Solid Edge part; units mm, degrees
sketch "Sketch1" plane through (0, 0, 0) normal (0, 0, 1) x (1, 0, 0)
  line L0 (-9, 9) -> (9, 9)
  line L1 (9, 9) -> (9, -9)
  line L2 (9, -9) -> (-9, -9)
  line L3 (-9, -9) -> (-9, 9)
  dimension "D1" = 9
  dimension "D2" = 9
extrude "Protrusion1" add sketch "Sketch1" along normal mid plane 6.5
sketch "Sketch2" plane through (0, 0, 3.25) normal (0, 0, 1) x (1, 0, 0)
  circle A0 centre (0, 0) radius 5
extrude "ExtrudedProtrusion_2" add sketch "Sketch2" along normal blind 75
chamfer "Chamfer_1" distance 1 angle 45 1 edges at (-5, 0, 78.25)
cosmetic_thread "Thread_1" thread depth 26
sketch "Sketch3" plane through (0, 0, 0) normal (1, 0, 0) x (0, 1, 0)
  line L0 (9, -3.25) -> (38.1568, 13.5837)
revolve "RevolvedCutout1" cut sketch "Sketch3" angle 360 about axis through (0, 0, -57) along (0, 0, 1) material side at (0, 23.6034, 5.1235)
Work out the finished part from the listing and answer in its coordinate system (mm). A direction names the side the tool comes from. Round coordinates to 2 decimals unless told otherwise and drop trailing zeros. Loops run counter-clockwise (first coordinate to the right, second up) from the corner with the lowest first, then second, coordinate; pieces in that order, holes last.
(1) Find the intervals of material crossed by L1, parallel to Z at x = -3.5, y = 6.25; L2, parallel to Y at x = -2, z = 41; L3, parallel to X at y = -1, z = 47.5, in increasing order.
Computed values:
L1: z = -3.25 to 3.25
L2: y = -4.58 to 4.58
L3: x = -4.9 to 4.9
(2) The part is cut by section A-A, the plane z = 43.5. Give the vertices of the cut face in (x, y).
Computed values:
outline: circle Ø10 at (0, 0)
(3) Each of these flat-tipped pins is pushed along its axis until it touches: P1, Ø2, axis at x = -6.5, y = 0, coming from the +Z side; P2, Ø1, axis at x = -1, z = 37, coming from the -Y side; P3, Ø4, axis at x = 1.5, y = -6, coming from the +Z side. Where does it stop, or does it pass through?
Computed values:
P1: stops at z = 3.25
P2: stops at y = -4.97
P3: stops at z = 78.07
(4) For faces 1 (the flat face through (4, -4, 3.25)), 2 (the flat face through (0, 9, 0)), determine the directions among +Z, -Z, +X, -X, +Y, -Y from which every point of the face is accessible in a straight line to the end or side of a thin tool.
Computed values:
face 1: +Z
face 2: +Z, -Z, +X, -X, +Y
